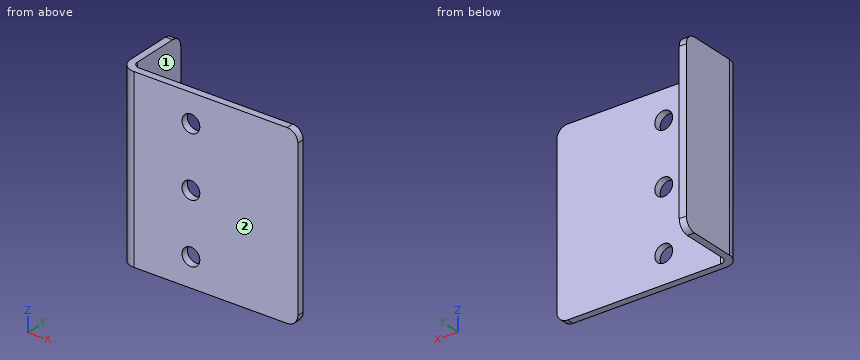
from build123d import *

# Parameters (mm, degrees)
SKETCH1_W                    = 50
SKETCH1_H                    = 50
BASE_FLANGE1_DEPTH           = 2
EDGE_FLANGE1_STRIP_W         = 12
EDGE_FLANGE1_STRIP_H         = 2
EDGE_FLANGE1_STRIP_CUT_DEPTH = 50
EDGE_FLANGE1_DEPTH           = 50
F_5_0MM_DOWEL_HOLE1_D        = 5
FILLET1_R                    = 3


# Sheet-metal steps are written as plain solids
with BuildPart() as part:
    # Sketch1 → Base-Flange1 (new body)
    with BuildSketch(Plane(origin=(0, 0, 0), x_dir=(1, 0, 0), z_dir=(0, 1, 0))):
        Rectangle(SKETCH1_W, SKETCH1_H)
    extrude(amount=BASE_FLANGE1_DEPTH)

    # Edge-Flange1 strip (across the edge) → Edge-Flange1 strip cut (cut)
    with BuildSketch(Plane(origin=(-25, 2, -25), x_dir=(1, 0, 0), z_dir=(0, 0, 1))):
        with Locations((-2, -1)):
            Rectangle(EDGE_FLANGE1_STRIP_W, EDGE_FLANGE1_STRIP_H)
    extrude(amount=EDGE_FLANGE1_STRIP_CUT_DEPTH, mode=Mode.SUBTRACT)

    # Edge-Flange1 section (across the edge) → Edge-Flange1 (add)
    with BuildSketch(Plane(origin=(-25, 2, -25), x_dir=(1, 0, 0), z_dir=(0, 0, 1))):
        with BuildLine():
            Line((0, 2), (0, 18))
            Line((0, 18), (2, 18))
            Line((2, 18), (2, 2))
            ThreePointArc((2, 2), (2.585786438, 0.585786438), (4, 0))
            Line((4, 0), (4, -2))
            ThreePointArc((4, -2), (1.171572875, -0.828427125), (0, 2))
        make_face()
    extrude(amount=EDGE_FLANGE1_DEPTH)

    # Ø5.0mm Dowel Hole1 (through all)
    with Locations(Plane(origin=(0, 2, 0), x_dir=(1, 0, 0), z_dir=(0, 1, 0))):
        with Locations((-5, 17), (-5, 0), (-5, -17)):
            Hole(F_5_0MM_DOWEL_HOLE1_D / 2)

    # Fillet1
    fillet1_edges = [part.edges().sort_by_distance(p)[0] for p in [
        (-24, 20, -25),
        (-24, 20, 25),
        (25, 1, -25),
        (25, 1, 25),
    ]]
    fillet(fillet1_edges, radius=FILLET1_R)


solid = part.part
The model under review builds one solid part; all positions refer to its coordinate system, in mm. Face numbers are marked on the shaded views. A direction names the side the tool comes from. Give positions to 0.01 mm unless a question says otherwise; leave off trailing zeros. Write each loop counter-clockwise with the first axis right and the second up, starting at its lowest first coordinate (ties: lowest second). Pieces come first, ordered by that corner, then holes.
1. Add section B-B, the plane x = -5. Write out the cut boundary in (y, z).
2. Add section C-C, the plane z = -6.5. Write out the cut boundary in (x, y).
3. Add section A-A, the plane z = 15.5. Write out the cut boundary in (x, y), plus the area to 3 significant figures.
4. Wall thickness on L1, parallel to Z at x = -5, y = 1.45; L2, parallel to X at y = 5.5, z = -17.5; L3, parallel to Y at x = 15, z = -4.5: over which ranges is each line inside the solid? List them lowest first.
5. For P1, Ø4, axis at x = -16.5, z = 0.5, coming from the +Y side; P2, Ø4, axis at x = -3.5, z = -1, coming from the -Y side; P3, Ø2, axis at y = 17.5, z = -2, coming from the +X side, all flat-tipped, find the tip position at first contact; note any pin that passes through.
6. Add section D-D, the plane y = 10.75. Write out the cut boundary in (x, z), plus the area to 3 significant figures.
7. Tool access review of the marked faces 1 and 2: name each direction out of +Z, -Z, +X, -X, +Y, -Y from which nothing blocks a thin tool from reaching the whole face with its end or side.
Worked answers:
1. outline: (0, -25) - (2, -25) - (2, -19.5) - (0, -19.5) - close; (0, -14.5) - (2, -14.5) - (2, -2.5) - (0, -2.5) - close; (0, 2.5) - (2, 2.5) - (2, 14.5) - (0, 14.5) - close; (0, 19.5) - (2, 19.5) - (2, 25) - (0, 25) - close
2. outline: (-25, 4) arc R4 ccw to (-21, 0) - (25, 0) - (25, 2) - (-21, 2) arc R2 cw to (-23, 4) - (-23, 20) - (-25, 20) - close
3. outline: (-25, 4) arc R4 ccw to (-21, 0) - (-7, 0) - (-7, 2) - (-21, 2) arc R2 cw to (-23, 4) - (-23, 20) - (-25, 20) - close; (-3, 0) - (25, 0) - (25, 2) - (-3, 2) - close
3. area: 125 mm2
4. L1: z = -25 to -19.5, -14.5 to -2.5, 2.5 to 14.5, 19.5 to 25
4. L2: x = -25 to -23
4. L3: y = 0 to 2
5. P1: stops at y = 2
5. P2: stops at y = 0
5. P3: stops at x = -23
6. outline: (-25, -25) - (-23, -25) - (-23, 25) - (-25, 25) - close
6. area: 100 mm2
7. face 1: +Z, -Z, +X, +Y
7. face 2: +Z, -Z, +X, -X, -Y
